Check sheet for the modelled part. Datum: model origin and axes. Units: mm. A direction names the side the tool comes from. Give positions to 0.01 mm unless a question says otherwise; leave off trailing zeros. Order: outer loops, then holes, each group sorted by start corner. A loop starts at its lowest first (then second) coordinate and runs counter-clockwise, first axis right, second up.
from build123d import *
from build123d.topology import SkipClean

# Parameters (mm, degrees)
CROQUIS1_R                    = 4.218255418
CROQUIS1_R_2                  = 4
SALIENTE_EXTRUIR1_DEPTH       = 1
SALIENTE_EXTRUIR2_START       = -4
SALIENTE_EXTRUIR2_OUTLINE_R   = 4.5
SALIENTE_EXTRUIR2_OUTLINE_R_2 = 4.218255418
SALIENTE_EXTRUIR2_DEPTH       = 6
CROQUIS3_R                    = 5
CROQUIS3_R_2                  = 4.218255418
SALIENTE_EXTRUIR3_DEPTH       = 0.5
CROQUIS4_R                    = 5.3
CROQUIS4_R_2                  = 4.5
SALIENTE_EXTRUIR5_DEPTH       = 0.1
CROQUIS5_R                    = 5.3
CROQUIS5_R_2                  = 5
SALIENTE_EXTRUIR6_DEPTH       = 6.337921


# Read off the part's stored shape, not the designer's step: Saliente-Extruir2
with BuildPart() as part:
    # Croquis1 → Saliente-Extruir1 (new body)
    with BuildSketch(Plane(origin=(0, 0, 0), x_dir=(1, 0, 0), z_dir=(0, 1, 0))):
        with BuildLine():
            ThreePointArc((3.313459582, 4.10165926), (-4.681239764, 2.42664735), (-1.441875065, -5.071845757))
            ThreePointArc((-1.441875065, -5.071845757), (8.628437932, -14.919813028), (5.858493799, -28.729993067))
            ThreePointArc((5.858493799, -28.729993067), (7.278526743, -36.308249114), (14.452018201, -33.482036353))
            ThreePointArc((14.452018201, -33.482036353), (14.728457578, -12.957711758), (3.313459582, 4.10165926))
        make_face()
        with Locations(Location((0, 0, 0), (0, 0, 270))):
            Circle(CROQUIS1_R, mode=Mode.SUBTRACT)
        with Locations(Location((9.698123587, -31.932686167, 0), (0, 0, 270))):
            Circle(CROQUIS1_R_2, mode=Mode.SUBTRACT)
    extrude(amount=SALIENTE_EXTRUIR1_DEPTH)

    # Saliente-Extruir2 outline → Saliente-Extruir2 (add)
    with SkipClean():  # the faces are left unmerged after this step: merging them gives an invalid solid
        with BuildSketch(Plane(origin=(0, 1, 0), x_dir=(1, 0, 0), z_dir=(0, 1, 0)).offset(SALIENTE_EXTRUIR2_START)):
            Circle(SALIENTE_EXTRUIR2_OUTLINE_R)
            Circle(SALIENTE_EXTRUIR2_OUTLINE_R_2, mode=Mode.SUBTRACT)
        extrude(amount=SALIENTE_EXTRUIR2_DEPTH)

    # Croquis3 → Saliente-Extruir3 (add)
    with BuildSketch(Plane(origin=(0, 3, 0), x_dir=(1, 0, 0), z_dir=(0, 1, 0))):
        with Locations(Location((0, 0, 0), (0, 0, 270))):
            Circle(CROQUIS3_R)
        with Locations(Location((0, 0, 0), (0, 0, 270))):
            Circle(CROQUIS3_R_2, mode=Mode.SUBTRACT)
    extrude(amount=SALIENTE_EXTRUIR3_DEPTH)

    # Croquis4 → Saliente-Extruir5 (add)
    with BuildSketch(Plane.XZ):
        with Locations(Location((9.698123587, 31.932686167, 0), (0, 0, 357.04362328))):
            Circle(CROQUIS4_R)
        with Locations(Location((9.698123587, 31.932686167, 0), (0, 0, 270))):
            Circle(CROQUIS4_R_2, mode=Mode.SUBTRACT)
    extrude(amount=SALIENTE_EXTRUIR5_DEPTH)

    # Croquis5 → Saliente-Extruir6 (add)
    with BuildSketch(Plane.XZ.offset(0.1)):
        with Locations(Location((9.698123587, 31.932686167, 0), (0, 0, 357.04362328))):
            Circle(CROQUIS5_R)
        with Locations(Location((9.698123587, 31.932686167, 0), (0, 0, 270))):
            Circle(CROQUIS5_R_2, mode=Mode.SUBTRACT)
    extrude(amount=SALIENTE_EXTRUIR6_DEPTH)


solid = part.part
1) Section check A-A, the plane z = 0. Record the cut outline in (x, y).
Recorded:
outline: (-5.27, 0) - (-4.5, 0) - (-4.5, -3) - (-4.22, -3) - (-4.22, 3.5) - (-5, 3.5) - (-5, 3) - (-4.5, 3) - (-4.5, 1) - (-5.27, 1) - close; (4.22, -3) - (4.5, -3) - (4.5, 0) - (7.58, 0) - (7.58, 1) - (4.5, 1) - (4.5, 3) - (5, 3) - (5, 3.5) - (4.22, 3.5) - close
2) Material ranges on L1, parallel to Z at x = 0, y = -0.25; L2, parallel to Z at x = 10, y = -0.5; L3, parallel to Y at x = 5.75, z = -1.5, recorded low to high.
Recorded:
L1: z = -4.5 to -4.22, 4.22 to 4.5
L2: z = 26.64 to 26.94, 36.92 to 37.22
L3: y = 0 to 1
3) Draft check along X on faces 4 (the face through (9.918, -3.225, 36.928)), 5 (the face through (8.566, 0.493, 14.724)), 6 (the face through (-4, 3.5, -2)). Enter one of: +X half, -X half, draft (parallel to the pull), parting line (faces both ways), or undercut.
Recorded:
face 4: undercut
face 5: -X half
face 6: draft
4) Section check D-D, the plane y = 1.75. Record the cut outline in (x, z).
Recorded:
outline: circle Ø9 at (0, 0); hole circle Ø8.44 at (0, 0)
5) Section check B-B, the plane x = 7.25. Record the cut outline in (y, z).
Recorded:
outline: (-6.44, 27.23) - (0, 27.23) - (0, 26.75) - (1, 26.75) - (1, 28.77) - (0, 28.77) - (0, 28.16) - (-0.1, 28.16) - (-0.1, 27.57) - (-6.44, 27.57) - close; (-6.44, 36.29) - (-0.1, 36.29) - (-0.1, 35.71) - (0, 35.71) - (0, 35.1) - (1, 35.1) - (1, 36.29) - (0, 36.29) - (0, 36.63) - (-6.44, 36.63) - close; (0, -0.37) - (1, -0.37) - (1, 11.79) - (0, 11.79) - close
6) Set-up check for faces 1 (the face through (-4.62, 0.49, -2.54)), 2 (the face through (-4.88, 3.25, -1.08)), 3 (the face through (6, 0, 34)): record each of +Z, -Z, +X, -X, +Y, -Y from which the full face is reachable in a straight line by a thin tool's end or side.
Recorded:
face 1: +Y, -Y
face 2: +Y
face 3: -Y
7) Depth check by flat-ended pin: pin 1 Ø2 at (y, z) = (-0.5, 23.5) entering from +X; pin 2 Ø4.5 at (x, z) = (2, 1.5) entering from -Y; pin 3 Ø5 at (x, z) = (11, 33.5) entering from -Y; pin 4 Ø11.5 at (x, z) = (9.7, 31.93) entering from +Y. Enter the tip coordinate at first touch or a pass-through.
Recorded:
pin 1: stops at x = 16.15
pin 2: stops at y = -3
pin 3: stops at y = -0.1
pin 4: stops at y = 1
8) Section check C-C, the plane x = 2. Record the cut outline in (y, z).
Recorded:
outline: (-3, -4.03) - (0, -4.03) - (0, -4.88) - (1, -4.88) - (1, -4.03) - (3, -4.03) - (3, -4.58) - (3.5, -4.58) - (3.5, -3.71) - (-3, -3.71) - close; (-3, 3.71) - (3.5, 3.71) - (3.5, 4.58) - (3, 4.58) - (3, 4.03) - (1, 4.03) - (1, 6.54) - (0, 6.54) - (0, 4.03) - (-3, 4.03) - close
